```python
from build123d import *

# Parameters (mm, degrees)
BOSS_EXTRUDE1_DEPTH = 10
SKETCH2_W           = 5
SKETCH2_H           = 25
CUT_EXTRUDE1_DEPTH  = 10
SKETCH3_R           = 1.25
CUT_EXTRUDE2_DEPTH  = 27.925824036
BOSS_EXTRUDE3_DEPTH = 20
SKETCH7_R           = 1.25
CUT_EXTRUDE3_DEPTH  = 20


with BuildPart() as part:
    # Sketch1 → Boss-Extrude1 (new, symmetric)
    with BuildSketch(Plane.XY):
        with BuildLine():
            Line((-10, -15), (10, -15))
            Line((10, -15), (10, 5))
            ThreePointArc((10, 5), (0, 15), (-10, 5))
            Line((-10, 5), (-10, -15))
        make_face()
    extrude(amount=BOSS_EXTRUDE1_DEPTH, both=True)

    # Sketch2 → Cut-Extrude1 (cut, symmetric)
    with BuildSketch(Plane(origin=(0, 0, 0), x_dir=(0, 0, -1), z_dir=(1, 0, 0))):
        with Locations((0, 2.5)):
            Rectangle(SKETCH2_W, SKETCH2_H)
    extrude(amount=CUT_EXTRUDE1_DEPTH, both=True, mode=Mode.SUBTRACT)

    # Sketch3 → Cut-Extrude2 (cut, through all)
    with BuildSketch(Plane.XY.offset(10)):
        with Locations((0, 5)):
            Circle(SKETCH3_R)
    extrude(amount=-CUT_EXTRUDE2_DEPTH, mode=Mode.SUBTRACT)

    # Sketch6 → Boss-Extrude3 (add)
    with BuildSketch(Plane(origin=(10, 0, 0), x_dir=(0, 0, -1), z_dir=(1, 0, 0))):
        with BuildLine():
            Line((-10, -15), (9.932520062, -15))
            ThreePointArc((9.932520062, -15), (-0.033739969, -24.966260031), (-10, -15))
        make_face()
    extrude(amount=-BOSS_EXTRUDE3_DEPTH)

    # Sketch7 → Cut-Extrude3 (cut)
    with BuildSketch(Plane(origin=(10, 0, 0), x_dir=(0, 0, -1), z_dir=(1, 0, 0))):
        with Locations((-0.033739969, -15)):
            Circle(SKETCH7_R)
    extrude(amount=-CUT_EXTRUDE3_DEPTH, mode=Mode.SUBTRACT)


solid = part.part
```
Could you check a few things on this model? Use its own coordinates, in mm. A direction names the side the tool comes from. Round coordinates to 2 decimals unless told otherwise and drop trailing zeros. Write each loop counter-clockwise with the first axis right and the second up, starting at its lowest first coordinate (ties: lowest second). Pieces come first, ordered by that corner, then holes. Notation, with made-up numbers: M 89.5,42 L 115.5,42 A19 cw 115.5,72 Z; hole C 54,47.5 d6. An arc over 180 degrees is marked long. Write each question's results on one line, items separated by ' | '. Start each with the question number.
1. I need wall thicknesses on L1, parallel to Z at x = -4, y = 0.5; L2, parallel to Z at x = 0.5, y = -14.5; L3, parallel to Y at x = 0, z = 5.25. Which ranges of each line are inside material? Lowest first, please. Write a range as from..to.
2. Imagine slicing it at C-C on z = -5.5. List the corners of the cut face in (x, y) for me, and give its area (3 significant figures).
3. Imagine slicing it at B-B on y = 3. List the corners of the cut face in (x, z) for me, and give its area (3 significant figures).
4. On a 3-axis mill with a long thin cutter (end or side, diameter ignored), from which of +Z, -Z, +X, -X, +Y, -Y can I reach the whole of each face in a straight line? I mean faces 1 (the face through (0, 15, -6)), 2 (the face through (0, 2, -2.5)). Say none if no direction works.
5. Thinking about a two-plate mould opening in X: for faces 3 (the face through (0.14, -13.76, 0.2)), 4 (the face through (-0.27, 3.78, -6.2)), 5 (the face through (-10, -13, 0)), which applies, +X half, -X half, draft (parallel to the pull), parting line (faces both ways), or undercut?
6. I'm going to push flat-ended pins straight in: pin 1 Ø4 at (x, z) = (0.5, 0) entering from +Y; pin 2 Ø3 at (x, z) = (7.5, -7) entering from +Y. Where does each tip first touch, or does it pass through?
Result sheet:
1) L1: z = -10..-2.5, 2.5..10 | L2: z = -10..-1.11, 1.18..10 | L3: y = -23.49..3.75, 6.25..15
2) outline: M -10,-23.29 L 10,-23.29 L 10,5 A10 ccw -10,5 Z; hole C 0,5 d2.5 | area: 718 mm^2
3) outline: M -10,-10 L 10,-10 L 10,-2.5 L -10,-2.5 Z; M -10,2.5 L 10,2.5 L 10,10 L -10,10 Z | area: 300 mm^2
4) face 1: +Z, -Z, +Y | face 2: +X, -X, +Y
5) face 3: draft | face 4: undercut | face 5: -X half
6) pin 1: stops at y = -10 | pin 2: stops at y = 13
